Geometry: final body of the model. Coordinates: model frame, mm. A direction names the side the tool comes from. Coordinates: 2 decimals unless noted, no trailing zeros. Write each loop counter-clockwise with the first axis right and the second up, starting at its lowest first coordinate (ties: lowest second). Pieces come first, ordered by that corner, then holes.
from build123d import *

# Parameters (mm, degrees)
SKETCH_1_W          = 51
SKETCH_1_H          = 79
EXTRUDE_1_DEPTH     = 28.8
SKETCH_2_R          = 1.5
CUT_EXTRUDE_1_DEPTH = 5
SKETCH_3_R          = 1.5
CUT_EXTRUDE_2_DEPTH = 5
SKETCH_4_W          = 41
SKETCH_4_H          = 12
CUT_EXTRUDE_3_DEPTH = 5


with BuildPart() as part:
    # 草图1 → 凸台-拉伸1 (new body)
    with BuildSketch(Plane.XY):
        Rectangle(SKETCH_1_W, SKETCH_1_H)
    extrude(amount=EXTRUDE_1_DEPTH)

    # 草图2 → 切除-拉伸1 (cut)
    with BuildSketch(Plane(origin=(0, 0, 0), x_dir=(-1, 0, 0), z_dir=(0, 0, -1))):
        with Locations((0, 29)):
            Circle(SKETCH_2_R)
        with Locations((0, -26)):
            Circle(SKETCH_2_R)
    extrude(amount=-CUT_EXTRUDE_1_DEPTH, mode=Mode.SUBTRACT)

    # 草图3 → 切除-拉伸2 (cut)
    with BuildSketch(Plane(origin=(25.5, 0, 0), x_dir=(0, 0, -1), z_dir=(1, 0, 0))):
        with Locations(Location((-14, 37.6, 0), (0, 0, 90))):
            Circle(SKETCH_3_R)
        with Locations(Location((-14, -28.9, 0), (0, 0, 90))):
            Circle(SKETCH_3_R)
    extrude(amount=-CUT_EXTRUDE_2_DEPTH, mode=Mode.SUBTRACT)

    # 草图4 → 切除-拉伸3 (cut)
    with BuildSketch(Plane.XZ.offset(39.5)):
        with Locations((-5, 11)):
            Rectangle(SKETCH_4_W, SKETCH_4_H)
    extrude(amount=-CUT_EXTRUDE_3_DEPTH, mode=Mode.SUBTRACT)


solid = part.part
Item 1: Pull-direction query (Z, two-part tool) for faces 1 (the cylindrical face through (23.04, -30.4, 14.07)), 2 (the flat face through (0, 29, 5)), 3 (the cylindrical face through (0.195, 30.487, 2.465)), 4 (the cylindrical face through (23.04, 36.1, 14.07)); classes: released by +Z, released by -Z, zero draft, split by the parting line, or undercut.
Derived:
face 1: undercut
face 2: released by -Z
face 3: zero draft
face 4: undercut
Item 2: Section B-B, the plane z = 14. Output: boundary loops of the cut face in (x, y), plus the area to 3 significant figures.
Derived:
outline: (-25.5, -34.5) - (15.5, -34.5) - (15.5, -39.5) - (25.5, -39.5) - (25.5, -30.4) - (20.5, -30.4) - (20.5, -27.4) - (25.5, -27.4) - (25.5, 36.1) - (20.5, 36.1) - (20.5, 39.1) - (25.5, 39.1) - (25.5, 39.5) - (-25.5, 39.5) - close
area: 3,790 mm2
Item 3: Pin query (flat end, axial travel): pin 1 (0.9 mm diameter, centred on y = -29.5, z = 13.5, fed in from +X). Return the tip coordinate at first contact, or that it passes through.
Derived:
pin 1: stops at x = 20.5
Item 4: Section D-D, the plane z = 10.5. Output: boundary loops of the cut face in (x, y).
Derived:
outline: (-25.5, -34.5) - (15.5, -34.5) - (15.5, -39.5) - (25.5, -39.5) - (25.5, 39.5) - (-25.5, 39.5) - close
Item 5: Material intervals for probe 1 along Y at (x, z) = (0, 3.3); probe 2 along Z at (x, y) = (23.55, -28.9); probe 3 along Y at (x, z) = (-7.5, 10), sorted ascending.
Derived:
probe 1: y = -39.5 to -27.5, -24.5 to 27.5, 30.5 to 39.5
probe 2: z = 0 to 12.5, 15.5 to 28.8
probe 3: y = -34.5 to 39.5
Item 6: Set-up query: faces 5 (the flat face through (0, 39.5, 14)), 6 (the flat face through (15.5, -37, 11)), 7 (the flat face through (0, -26, 5)), 8 (the flat face through (20.5, -29, 14)). Return all of +Z, -Z, +X, -X, +Y, -Y with unobstructed straight access to the full face (end or side cutting, diameter ignored); none if empty.
Derived:
face 5: +Z, -Z, +X, -X, +Y
face 6: -X, -Y
face 7: -Z
face 8: +X
Item 7: Section A-A, the plane x = -6. Output: boundary loops of the cut face in (y, z), plus the area to 3 significant figures.
Derived:
outline: (-39.5, 0) - (39.5, 0) - (39.5, 28.8) - (-39.5, 28.8) - (-39.5, 17) - (-34.5, 17) - (-34.5, 5) - (-39.5, 5) - close
area: 2,220 mm2
Item 8: Section C-C, the plane x = 0. Output: boundary loops of the cut face in (y, z), plus the area to 3 significant figures.
Derived:
outline: (-39.5, 0) - (-27.5, 0) - (-27.5, 5) - (-24.5, 5) - (-24.5, 0) - (27.5, 0) - (27.5, 5) - (30.5, 5) - (30.5, 0) - (39.5, 0) - (39.5, 28.8) - (-39.5, 28.8) - (-39.5, 17) - (-34.5, 17) - (-34.5, 5) - (-39.5, 5) - close
area: 2,190 mm2
